Input: part model. Units: mm. Frame: model coordinates. Give positions to 0.01 mm unless a question says otherwise; leave off trailing zeros. Write each loop counter-clockwise with the first axis right and the second up, starting at its lowest first coordinate (ties: lowest second). Pieces come first, ordered by that corner, then holes. Notation, with made-up numbers: (16, -15.75) - (43, -15.75) arc R13 cw to (43, -7.75) - close; hole circle Ø9 at (83.5, 62). An arc over 180 degrees is marked (long way). Answer as CSV lines item,"result". Start each with the question number.
from build123d import *

# Parameters (mm, degrees)
SKETCH2_R           = 1.5
BOSS_EXTRUDE2_DEPTH = 3


with BuildPart() as part:
    # Sketch2 → Boss-Extrude2 (new body)
    with BuildSketch(Plane(origin=(0, 0, 0), x_dir=(1, 0, 0), z_dir=(0, 1, 0))):
        with BuildLine():
            Line((0, 4), (80, 4))
            ThreePointArc((80, 4), (84, 0), (80, -4))
            Line((80, -4), (0, -4))
            ThreePointArc((0, -4), (-4, 0), (0, 4))
        make_face()
        with Locations(Location((0, 0, 0), (0, 0, 270))):
            Circle(SKETCH2_R, mode=Mode.SUBTRACT)
        with Locations(Location((8, 0, 0), (0, 0, 270))):
            Circle(SKETCH2_R, mode=Mode.SUBTRACT)
        with Locations(Location((16, 0, 0), (0, 0, 270))):
            Circle(SKETCH2_R, mode=Mode.SUBTRACT)
        with Locations(Location((24, 0, 0), (0, 0, 270))):
            Circle(SKETCH2_R, mode=Mode.SUBTRACT)
        with Locations(Location((32, 0, 0), (0, 0, 270))):
            Circle(SKETCH2_R, mode=Mode.SUBTRACT)
        with Locations(Location((40, 0, 0), (0, 0, 270))):
            Circle(SKETCH2_R, mode=Mode.SUBTRACT)
        with Locations(Location((48, 0, 0), (0, 0, 270))):
            Circle(SKETCH2_R, mode=Mode.SUBTRACT)
        with Locations(Location((56, 0, 0), (0, 0, 270))):
            Circle(SKETCH2_R, mode=Mode.SUBTRACT)
        with Locations(Location((64, 0, 0), (0, 0, 270))):
            Circle(SKETCH2_R, mode=Mode.SUBTRACT)
        with Locations(Location((72, 0, 0), (0, 0, 270))):
            Circle(SKETCH2_R, mode=Mode.SUBTRACT)
        with Locations(Location((80, 0, 0), (0, 0, 270))):
            Circle(SKETCH2_R, mode=Mode.SUBTRACT)
    extrude(amount=BOSS_EXTRUDE2_DEPTH)


solid = part.part
1) Contact query for flat-ended pins moving along their axis: P1, Ø1.8, axis at x = 32, z = 0, coming from the +Y side; P2, Ø1.5, axis at y = 2.5, z = 1, coming from the +X side. Output: stop coordinate, or through.
2) Cut plane D-D on z = -3.25. Output: boundary loops of the cut face in (x, y).
3) Cut plane A-A on x = 40. Output: boundary loops of the cut face in (y, z).
4) Pull-direction query (X, two-part tool) for faces 1 (the cylindrical face through (65.265, 1.479, 0.806)), 2 (the cylindrical face through (0.45, 1.48, 1.43)), 3 (the flat face through (39, 1, -4)), 4 (the cylindrical face through (84, 1, 0)); classes: +X half, -X half, draft (parallel to the pull), parting line (faces both ways), or undercut.
5) Cut plane B-B on y = 1.35. State how many separate pieces and enclosed holes the cut face has, and give its area (3 significant figures).
6) Material intervals for line 1 (Z direction, x = 39, y = 2.05); line 2 (Z direction, x = 40.5, y = 0.65); line 3 (X direction, y = 1.45, z = -2.75), sorted ascending. Write a range as from..to.
Numbers:
1,P1,"passes through"
1,P2,"stops at x = 83.99"
2,outline,"(-2.33, 0) - (82.33, 0) - (82.33, 3) - (-2.33, 3) - close"
3,outline,"(0, -4) - (3, -4) - (3, -1.5) - (0, -1.5) - close; (0, 1.5) - (3, 1.5) - (3, 4) - (0, 4) - close"
4,face 1,"undercut"
4,face 2,"undercut"
4,face 3,"draft"
4,face 4,"+X half"
5,separate pieces,"1"
5,enclosed holes,"11"
5,area,"613 mm²"
6,line 1,"z = -4..-1.12, 1.12..4"
6,line 2,"z = -4..-1.41, 1.41..4"
6,line 3,"x = -2.9..82.9"
